```python
from build123d import *

# Parameters (mm, degrees)
EXTRUDE_1_DEPTH     = 18
HOLE_WIZARD_M6_1_D  = 5
SKETCH_7_R          = 3
CUT_EXTRUDE_1_DEPTH = 259.015029546
HOLE_WIZARD_M6_2_D  = 5


with BuildPart() as part:
    # 草图1 → 凸台-拉伸1 (new body)
    with BuildSketch(Plane.XY):
        Polygon((0, 0), (80, 0), (80, 60), (22.986425339, 129.63800905), (22.986425339, 244.63800905), (-47.013574661, 244.63800905), (-47.013574661, 104.63800905), (0, 47.214285714), align=None)
    extrude(amount=EXTRUDE_1_DEPTH)

    # M6 螺纹孔1 (through all)
    with Locations(Plane.XY.offset(18)):
        with Locations((-40.013574661, 114.63800905), (-22.013574661, 114.63800905), (-40.013574661, 234.63800905), (-22.013574661, 234.63800905)):
            Hole(HOLE_WIZARD_M6_1_D / 2)

    # 草图7 → 切除-拉伸1 (cut, through all)
    with BuildSketch(Plane.XY.offset(18)):
        with Locations((15, 15)):
            Circle(SKETCH_7_R)
        with Locations((40, 15)):
            Circle(SKETCH_7_R)
        with Locations((65, 15)):
            Circle(SKETCH_7_R)
    extrude(amount=-CUT_EXTRUDE_1_DEPTH, mode=Mode.SUBTRACT)

    # M6 螺纹孔2 (through all)
    with Locations(Plane(origin=(-42.013574661, 174.63800905, 18), x_dir=(1, 0, 0), z_dir=(0, 0, 1))):
        with Locations((0, 0)):
            Hole(HOLE_WIZARD_M6_2_D / 2)


solid = part.part
```
Input: part model. Units: mm. Frame: model coordinates. A direction names the side the tool comes from. Give positions to 0.01 mm unless a question says otherwise; leave off trailing zeros. Order: outer loops, then holes, each group sorted by start corner. A loop starts at its lowest first (then second) coordinate and runs counter-clockwise, first axis right, second up. Notation, with made-up numbers: M -23,76.25 L 33,76.25 A19 cw 33,96.25 Z; hole C -23,-2 d2. An arc over 180 degrees is marked long. Return JSON: item names as keys, results as strings.
1) Section query D-D on x = 65.5. Output: boundary loops of the cut face in (y, z).
Taken from the geometry:
{"outline": "M 0,0 L 12.04,0 L 12.04,18 L 0,18 Z; M 17.96,0 L 77.71,0 L 77.71,18 L 17.96,18 Z"}
2) Section query A-A on x = 15. Output: boundary loops of the cut face in (y, z).
Taken from the geometry:
{"outline": "M 0,0 L 12,0 L 12,18 L 0,18 Z; M 18,0 L 244.64,0 L 244.64,18 L 18,18 Z"}
3) Section query B-B on y = 15. Output: boundary loops of the cut face in (x, z).
Taken from the geometry:
{"outline": "M 0,0 L 12,0 L 12,18 L 0,18 Z; M 18,0 L 37,0 L 37,18 L 18,18 Z; M 43,0 L 62,0 L 62,18 L 43,18 Z; M 68,0 L 80,0 L 80,18 L 68,18 Z"}
4) Access query for faces 1 (the face through (0, 24, 9)), 2 (the face through (12.6, 13.2, 9.1)), 3 (the face through (22.986, 186, 9)). Directions: +Z, -Z, +X, -X, +Y, -Y. A direction counts if a zero-diameter tool reaches every point of the face in a straight line with its end or side. Return the directions, or none.
Taken from the geometry:
{"face 1": "+Z, -Z, -X, -Y", "face 2": "+Z, -Z", "face 3": "+Z, -Z, +X, +Y"}
5) Mould query, pull axis Y, two halves, no side actions, for faces 4 (the face through (62.6, 13.2, 9.1)), 5 (the face through (-23.84, 76.33, 8.87)), 6 (the face through (-47.014, 176, 9)). Classes: released by +Y, released by -Y, zero draft, split by the parting line, or undercut.
Taken from the geometry:
{"face 4": "undercut", "face 5": "released by -Y", "face 6": "zero draft"}
6) Line query: L1, parallel to Y at x = 15, z = 11.5; L2, parallel to X at y = 186.5, z = 10.5; L3, parallel to Y at x = 65, z = 9.5. Output: solid intervals per line, ascending. Write a range as [from, to].
Taken from the geometry:
{"L1": "y = [0, 12], [18, 244.64]", "L2": "x = [-47.01, 22.99]", "L3": "y = [0, 12], [18, 78.32]"}
7) Contact query for flat-ended pins moving along their axis: pin 1 (6 mm diameter, centred on y = 203.5, z = 12, fed in from +X); pin 2 (1.5 mm diameter, centred on x = -16, z = 3.5, fed in from -Y). Output: stop coordinate, or through.
Taken from the geometry:
{"pin 1": "stops at x = 22.99", "pin 2": "stops at y = 65.84"}
8) Section query C-C on z = 5.75. Count the separate pieces of the cut face and the enclosed holes in it, and give its area (3 significant figures).
Taken from the geometry:
{"separate pieces": "1", "enclosed holes": "8", "area": "18,800 mm2"}
